Can you work these out from the model? Positions are in its coordinate system, mm. Coordinates: 2 decimals unless noted, no trailing zeros. Write each loop counter-clockwise with the first axis right and the second up, starting at its lowest first coordinate (ties: lowest second). Pieces come first, ordered by that corner, then holes. Notation, with made-up numbers: (48.25, 30.25) -> (56.25, 30.25) arc R14 ccw to (56.25, 51.25) -> close; hole circle Ø10 at (64.5, 55). An arc over 180 degrees is marked (long way). Use one line per item in the form item = value.
```python
from build123d import *

# Parameters (mm, degrees)
SKETCH_1_W          = 1500
SKETCH_1_H          = 2500
EXTRUDE_1_DEPTH     = 3
SKETCH_3_W          = 120
SKETCH_3_H          = 105
CUT_EXTRUDE_2_DEPTH = 2916.47749091
SKETCH_4_R          = 25
CUT_EXTRUDE_3_DEPTH = 300


with BuildPart() as part:
    # 草圖1 → 填料-伸長1 (new body)
    with BuildSketch(Plane.XY):
        with Locations((750, -1250)):
            Rectangle(SKETCH_1_W, SKETCH_1_H)
    extrude(amount=EXTRUDE_1_DEPTH)

    # 草圖3 → 除料-伸長2 (cut, through all)
    with BuildSketch(Plane.XY.offset(3)):
        with Locations((750, -1397.5)):
            Rectangle(SKETCH_3_W, SKETCH_3_H)
    extrude(amount=-CUT_EXTRUDE_2_DEPTH, mode=Mode.SUBTRACT)

    # 草圖4 → 除料-伸長3 (cut)
    with BuildSketch(Plane.XY.offset(3)):
        with Locations((1085.367901205, -1300)):
            Circle(SKETCH_4_R)
    extrude(amount=-CUT_EXTRUDE_3_DEPTH, mode=Mode.SUBTRACT)


solid = part.part
```
Q1. Thinking about a two-plate mould opening in Y: for faces 1 (the flat face through (740, -1232, 0)), 2 (the cylindrical face through (1096.9, -1322.18, 1.52)), which applies, released by +Y, released by -Y, zero draft, split by the parting line, or undercut?
Return value:
face_1 = zero draft
face_2 = undercut
Q2. If I drill on line 1 (X direction, y = -1300, z = 1.9); line 2 (X direction, y = -1416, z = 1.6); line 3 (Y direction, x = 733.5, z = 0.35), over which ranges is the centre line in solid material (lowest first)? Write a range as from..to.
Return value:
line_1 = 0..1060.37, 1110.37..1500
line_2 = 0..690, 810..1500
line_3 = -2500..-1450, -1345..0
Q3. Suppose I cut it at A-A (y = -1421.5). Write out the boundary of the cut face in (x, z).
Return value:
outline = (0, 0) -> (690, 0) -> (690, 3) -> (0, 3) -> close; (810, 0) -> (1500, 0) -> (1500, 3) -> (810, 3) -> close
